Here's how the part is built. I have some questions about the finished solid (model axes, mm). A direction names the side the tool comes from. Round coordinates to 2 decimals unless told otherwise and drop trailing zeros. Loops run counter-clockwise (first coordinate to the right, second up) from the corner with the lowest first, then second, coordinate; pieces in that order, holes last. Notation, with made-up numbers: M 29,20 L 68,20 A27 ccw 68,47 Z; hole C 29,9 d3. An arc over 180 degrees is marked long. Use a Markdown table: item, result.
from build123d import *

# Parameters (mm, degrees)
SKETCH1_W           = 50
SKETCH1_H           = 50
SKETCH1_W_2         = 2.5
SKETCH1_H_2         = 11.8
SKETCH1_W_3         = 2
SKETCH1_H_3         = 7
BOSS_EXTRUDE1_DEPTH = 2
SKETCH3_W           = 5
SKETCH3_H           = 2
CUT_EXTRUDE1_DEPTH  = 2
SKETCH4_W           = 5
SKETCH4_H           = 10
CUT_EXTRUDE2_DEPTH  = 2
CUT_EXTRUDE3_DEPTH  = 2


with BuildPart() as part:
    # Sketch1 → Boss-Extrude1 (new body)
    # profile 1 of 7: a face of its own
    with BuildSketch(Plane(origin=(0, 0, 0), x_dir=(1, 0, 0), z_dir=(0, 1, 0))):
        Rectangle(SKETCH1_W, SKETCH1_H)
        with Locations((15.75, 0.6)):
            Rectangle(SKETCH1_W_2, SKETCH1_H_2, mode=Mode.SUBTRACT)
    # profile 2 of 7: a face of its own
    with BuildSketch(Plane(origin=(0, 0, 0), x_dir=(1, 0, 0), z_dir=(0, 1, 0))):
        with Locations((26, 0)):
            Rectangle(SKETCH1_W_3, SKETCH1_H_3)
    # profile 3 of 7: a face of its own
    with BuildSketch(Plane(origin=(0, 0, 0), x_dir=(1, 0, 0), z_dir=(0, 1, 0))):
        with Locations((26, 15.5)):
            Rectangle(SKETCH1_W_3, SKETCH1_H_3)
    # profile 4 of 7: a face of its own
    with BuildSketch(Plane(origin=(0, 0, 0), x_dir=(1, 0, 0), z_dir=(0, 1, 0))):
        with Locations((26, -15.5)):
            Rectangle(SKETCH1_W_3, SKETCH1_H_3)
    # profile 5 of 7: a face of its own
    with BuildSketch(Plane(origin=(0, 0, 0), x_dir=(1, 0, 0), z_dir=(0, 1, 0))):
        with Locations((-26, 0)):
            Rectangle(SKETCH1_W_3, SKETCH1_H_3)
    # profile 6 of 7: a face of its own
    with BuildSketch(Plane(origin=(0, 0, 0), x_dir=(1, 0, 0), z_dir=(0, 1, 0))):
        with Locations((-26, -15.5)):
            Rectangle(SKETCH1_W_3, SKETCH1_H_3)
    # profile 7 of 7: a face of its own
    with BuildSketch(Plane(origin=(0, 0, 0), x_dir=(1, 0, 0), z_dir=(0, 1, 0))):
        with Locations((-26, 15.5)):
            Rectangle(SKETCH1_W_3, SKETCH1_H_3)
    extrude(amount=BOSS_EXTRUDE1_DEPTH)

    # Sketch3 → Cut-Extrude1 (cut)
    with BuildSketch(Plane(origin=(0, 2, 0), x_dir=(1, 0, 0), z_dir=(0, 1, 0))):
        with Locations((17.5, 24)):
            Rectangle(SKETCH3_W, SKETCH3_H)
        with Locations((17.5, -24)):
            Rectangle(SKETCH3_W, SKETCH3_H)
        with Locations((-17.5, 24)):
            Rectangle(SKETCH3_W, SKETCH3_H)
        with Locations((-17.5, -24)):
            Rectangle(SKETCH3_W, SKETCH3_H)
    extrude(amount=-CUT_EXTRUDE1_DEPTH, mode=Mode.SUBTRACT)

    # Sketch4 → Cut-Extrude2 (cut)
    with BuildSketch(Plane(origin=(0, 2, 0), x_dir=(1, 0, 0), z_dir=(0, 1, 0))):
        with Locations((3, 0)):
            Rectangle(SKETCH4_W, SKETCH4_H)
    extrude(amount=-CUT_EXTRUDE2_DEPTH, mode=Mode.SUBTRACT)

    # Sketch5 → Cut-Extrude3 (cut)
    with BuildSketch(Plane(origin=(0, 2, 0), x_dir=(1, 0, 0), z_dir=(0, 1, 0))):
        Polygon((-14.056788221, 16.417088801), (-8.5488143, 12.097109255), (-9.78309417, 10.52340242), (-15.291068091, 14.843381966), align=None)
    extrude(amount=-CUT_EXTRUDE3_DEPTH, mode=Mode.SUBTRACT)


solid = part.part
1. Imagine slicing it at C-C, the plane z = 6. Write out the boundary of the cut face in (x, y).
Answer sheet:
| item | result |
|---|---|
| outline | M -25,0 L 25,0 L 25,2 L -25,2 Z |
2. We'd pull the mould along Z, two halves only. Please class faces 5 (the face through (-15, 1, 24)), 6 (the face through (-26, 1, -19)), 7 (the face through (25, 1, -8)): +Z half, -Z half, draft (parallel to the pull), parting line (faces both ways), or undercut.
Answer sheet:
| item | result |
|---|---|
| face 5 | draft |
| face 6 | -Z half |
| face 7 | undercut |
3. I need wall thicknesses on probe 1 along Z at (x, y) = (2, 1.65); probe 2 along X at (y, z) = (0.7, 2.5); probe 3 along X at (y, z) = (1.85, 21). Which ranges of each line are inside material? Lowest first, please. Write a range as from..to.
Answer sheet:
| item | result |
|---|---|
| probe 1 | -25..-5, 5..25 |
| probe 2 | -27..0.5, 5.5..14.5, 17..27 |
| probe 3 | -25..25 |
4. Imagine slicing it at B-B, the plane y = 0.35. State how many separate pieces and enclosed holes the cut face has, then the cut area to 3 significant figures.
Answer sheet:
| item | result |
|---|---|
| separate pieces | 1 |
| enclosed holes | 3 |
| area | 2,450 mm2 |
5. Imagine slicing it at A-A, the plane z = -13.5. Write out the boundary of the cut face in (x, y).
Answer sheet:
| item | result |
|---|---|
| outline | M -27,0 L -13.58,0 L -13.58,2 L -27,2 Z; M -10.34,0 L 27,0 L 27,2 L -10.34,2 Z |
6. For pin 1 Ø10 at (x, z) = (8.5, -11.5) entering from -Y; pin 2 Ø0.6 at (x, y) = (15.5, 1) entering from -Z; pin 3 Ø0.6 at (y, z) = (1, -24) entering from +X; pin 4 Ø0.6 at (y, z) = (1, 24) entering from -X, each with a flat end and sliding along its axis, tell me the tip position at first contact or that it passes through.
Answer sheet:
| item | result |
|---|---|
| pin 1 | y = 0 |
| pin 2 | z = -23 |
| pin 3 | x = 25 |
| pin 4 | x = -25 |
7. Which directions (+Z, -Z, +X, -X, +Y, -Y) give clear straight access to the entire face, cutting with the end or side of a thin tool? Please do faces 1 (the face through (-9.16, 1.01, -11.32)), 2 (the face through (26, 1, -12)), 3 (the face through (17, 1, -23)), 4 (the face through (-26, 1, 3.5)).
Answer sheet:
| item | result |
|---|---|
| face 1 | +Y, -Y |
| face 2 | +X, +Y, -Y |
| face 3 | -Z, +Y, -Y |
| face 4 | -X, +Y, -Y |
